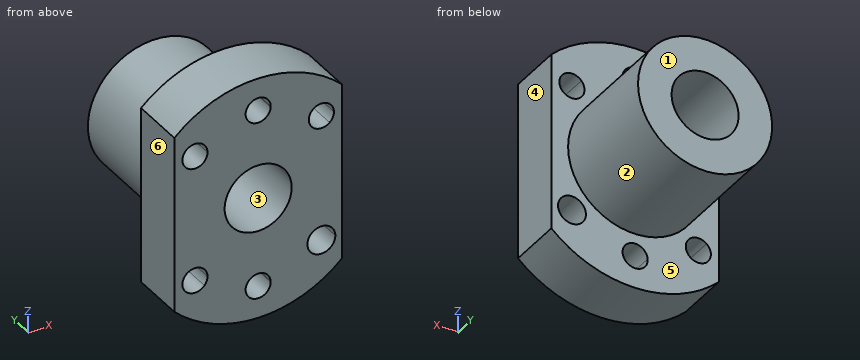
from build123d import *

# Parameters (mm, degrees)
SKETCH_1_R      = 6
EXTRUDE_1_DEPTH = 10
SKETCH_3_R      = 12
SKETCH_3_R_2    = 6
EXTRUDE_2_DEPTH = 21


with BuildPart() as part:
    # 草图1 → 凸台-拉伸1 (new body)
    with BuildSketch(Plane(origin=(0, 0, 0), x_dir=(1, 0, 0), z_dir=(0, 1, 0))):
        with BuildLine():
            ThreePointArc((-12.788894575, 9.614789418), (-14.041020916, 7.671357874), (-15, 5.567764363))
            Line((-15, 5.567764363), (-15, -5.567764363))
            ThreePointArc((-15, -5.567764363), (-14.041020916, -7.671357874), (-12.788894575, -9.614789418))
            ThreePointArc((-12.788894575, -9.614789418), (-10.380078131, -9.26655576), (-9.063708499, -11.313708499))
            ThreePointArc((-9.063708499, -11.313708499), (-9.205976551, -12.101087718), (-9.614789418, -12.788894575))
            ThreePointArc((-9.614789418, -12.788894575), (-6.122934918, -14.78207252), (-2.24443128, -15.841796875))
            ThreePointArc((-2.24443128, -15.841796875), (0, -13.75), (2.24443128, -15.841796875))
            ThreePointArc((2.24443128, -15.841796875), (6.122934918, -14.78207252), (9.614789418, -12.788894575))
            ThreePointArc((9.614789418, -12.788894575), (9.722718241, -9.722718241), (12.788894575, -9.614789418))
            ThreePointArc((12.788894575, -9.614789418), (14.041020916, -7.671357874), (15, -5.567764363))
            Line((15, -5.567764363), (15, 5.567764363))
            ThreePointArc((15, 5.567764363), (14.100687822, 7.561124451), (12.937965605, 9.413237806))
            ThreePointArc((12.937965605, 9.413237806), (9.545941546, 9.545941546), (9.413237806, 12.937965605))
            ThreePointArc((9.413237806, 12.937965605), (6.006943578, 14.829586267), (2.24443128, 15.841796875))
            ThreePointArc((2.24443128, 15.841796875), (0, 13.75), (-2.24443128, 15.841796875))
            ThreePointArc((-2.24443128, 15.841796875), (-6.122934918, 14.78207252), (-9.614789418, 12.788894575))
            ThreePointArc((-9.614789418, 12.788894575), (-9.205976551, 12.101087718), (-9.063708499, 11.313708499))
            ThreePointArc((-9.063708499, 11.313708499), (-10.380078131, 9.26655576), (-12.788894575, 9.614789418))
        make_face()
        Circle(SKETCH_1_R, mode=Mode.SUBTRACT)
        with BuildLine():
            Line((-15, -5.567764363), (-15, -15.84625977))
            ThreePointArc((-15, -15.84625977), (0, -21.819806339), (15, -15.84625977))
            Line((15, -15.84625977), (15, -5.567764363))
            ThreePointArc((15, -5.567764363), (14.041020916, -7.671357874), (12.788894575, -9.614789418))
            ThreePointArc((12.788894575, -9.614789418), (13.360861238, -10.380078131), (13.563708499, -11.313708499))
            ThreePointArc((13.563708499, -11.313708499), (12.101087718, -13.421440447), (9.614789418, -12.788894575))
            ThreePointArc((9.614789418, -12.788894575), (6.122934918, -14.78207252), (2.24443128, -15.841796875))
            ThreePointArc((2.24443128, -15.841796875), (2.248607389, -15.920849448), (2.25, -16))
            ThreePointArc((2.25, -16), (-0.079150552, -18.248607389), (-2.24443128, -15.841796875))
            ThreePointArc((-2.24443128, -15.841796875), (-6.122934918, -14.78207252), (-9.614789418, -12.788894575))
            ThreePointArc((-9.614789418, -12.788894575), (-12.904698757, -12.904698757), (-12.788894575, -9.614789418))
            ThreePointArc((-12.788894575, -9.614789418), (-14.041020916, -7.671357874), (-15, -5.567764363))
        make_face()
        with BuildLine():
            ThreePointArc((15, 15.84625977), (0, 21.819806339), (-15, 15.84625977))
            Line((-15, 15.84625977), (-15, 5.567764363))
            ThreePointArc((-15, 5.567764363), (-14.041020916, 7.671357874), (-12.788894575, 9.614789418))
            ThreePointArc((-12.788894575, 9.614789418), (-12.904698757, 12.904698757), (-9.614789418, 12.788894575))
            ThreePointArc((-9.614789418, 12.788894575), (-6.122934918, 14.78207252), (-2.24443128, 15.841796875))
            ThreePointArc((-2.24443128, 15.841796875), (-0.079150552, 18.248607389), (2.25, 16))
            ThreePointArc((2.25, 16), (2.248607389, 15.920849448), (2.24443128, 15.841796875))
            ThreePointArc((2.24443128, 15.841796875), (6.006943578, 14.829586267), (9.413237806, 12.937965605))
            ThreePointArc((9.413237806, 12.937965605), (12.179394143, 13.659041816), (13.813708499, 11.313708499))
            ThreePointArc((13.813708499, 11.313708499), (13.584241781, 10.267439596), (12.937965605, 9.413237806))
            ThreePointArc((12.937965605, 9.413237806), (14.100687822, 7.561124451), (15, 5.567764363))
            Line((15, 5.567764363), (15, 15.84625977))
        make_face()
    extrude(amount=EXTRUDE_1_DEPTH)

    # 草图3 → 凸台-拉伸2 (add)
    with BuildSketch(Plane(origin=(0, 10, 0), x_dir=(1, 0, 0), z_dir=(0, 1, 0))):
        Circle(SKETCH_3_R)
        Circle(SKETCH_3_R_2, mode=Mode.SUBTRACT)
    extrude(amount=EXTRUDE_2_DEPTH)


solid = part.part
Here's how the part is built. I have some questions about the finished solid (model axes, mm). Face numbers are marked on the shaded views. A direction names the side the tool comes from. Round coordinates to 2 decimals unless told otherwise and drop trailing zeros. Loops run counter-clockwise (first coordinate to the right, second up) from the corner with the lowest first, then second, coordinate; pieces in that order, holes last. Notation, with made-up numbers: M 10.25,-34 L 55.25,-34 A14 ccw 55.25,-25 Z; hole C 49,29 d10. An arc over 180 degrees is marked long. Write each question's results on one line, items separated by ' | '. Start each with the question number.
(1) I want a section at A-A (y = 5). Please give me the cut outline in (x, z), then the cut area to 3 significant figures.
(2) On a 3-axis mill with a long thin cutter (end or side, diameter ignored), from which of +Z, -Z, +X, -X, +Y, -Y can I reach the whole of each face in a straight line? I mean the marked faces 5 and 6. Say none if no direction works.
(3) I want a section at B-B (x = 0). Please give me the cut outline in (y, z).
(4) I want a section at C-C (z = 0). Please give me the cut outline in (x, y).
(5) I want a section at D-D (x = 5.5). Please give me the cut outline in (y, z).
(6) Thinking about a two-plate mould opening in X: for the marked faces 1, 2, 3 and 4, which applies, pulls with the +X half, pulls with the -X half, needs draft (parallel to the pull), parting line crosses it, or undercut?
(7) If I drill on probe 1 along Z at (x, y) = (0, 21.5); probe 2 along Z at (x, y) = (12, 2), over which ranges is the centre line in solid material (lowest first)? Write a range as from..to.
(8) Will these pins go through, and if not, where does the flat tip stop? P1, Ø1.5, axis at x = 5.5, y = 5.5, coming from the -Z side; P2, Ø8, axis at x = 7, y = 22.5, coming from the +Z side; P3, Ø5, axis at x = -9.5, z = 6.5, coming from the -Y side; P4, Ø4, axis at x = 6, y = 27, coming from the -Z side.
Solved:
1) outline: M -15,-15.85 A21.82 ccw 15,-15.85 L 15,15.85 A21.82 ccw -15,15.85 Z; hole C -11.31,-11.31 d4.5; hole C -11.31,11.31 d4.5; hole C 0,0 d12; hole C 0,-16 d4.5; hole C 0,16 d4.5; hole C 11.31,-11.31 d5; hole C 11.31,11.31 d4.5 | area: 985 mm²
2) face 5: +Y | face 6: +Z, -Z, -X, +Y, -Y
3) outline: M 0,-21.82 L 10,-21.82 L 10,-18.25 L 0,-18.25 Z; M 0,-13.75 L 10,-13.75 L 10,-12 L 31,-12 L 31,-6 L 0,-6 Z; M 0,6 L 31,6 L 31,12 L 10,12 L 10,13.75 L 0,13.75 Z; M 0,18.25 L 10,18.25 L 10,21.82 L 0,21.82 Z
4) outline: M -15,0 L -6,0 L -6,31 L -12,31 L -12,10 L -15,10 Z; M 6,0 L 15,0 L 15,10 L 12,10 L 12,31 L 6,31 Z
5) outline: M 0,-21.12 L 10,-21.12 L 10,-10.67 L 31,-10.67 L 31,-2.4 L 0,-2.4 Z; M 0,2.4 L 31,2.4 L 31,10.67 L 10,10.67 L 10,21.12 L 0,21.12 Z
6) face 1: needs draft | face 2: parting line crosses it | face 3: undercut | face 4: pulls with the +X half
7) probe 1: z = -12..-6, 6..12 | probe 2: z = -18.22..-13.72, -8.91..9.17, 13.46..18.22
8) P1: stops at z = -21.3 | P2: stops at z = 11.62 | P3: stops at y = 0 | P4: stops at z = -11.31
